Answer from the drawing. Dimensions are ordinates in mm from the lowest x, y and z of the part. Round coordinates to 2 decimals unless told otherwise and drop trailing zeros. Write each loop counter-clockwise with the first axis right and the second up, starting at its lowest first coordinate (ties: lowest second). Pieces come first, ordered by that corner, then holes. Notation, with made-up numbers: (69.25, -5.5) - (93.25, -5.5) arc R35 ccw to (93.25, 27.5) - close; hole circle Ø10 at (81, 62). An arc over 180 degrees is marked (long way). Answer as a JSON object with one key per item and string values.
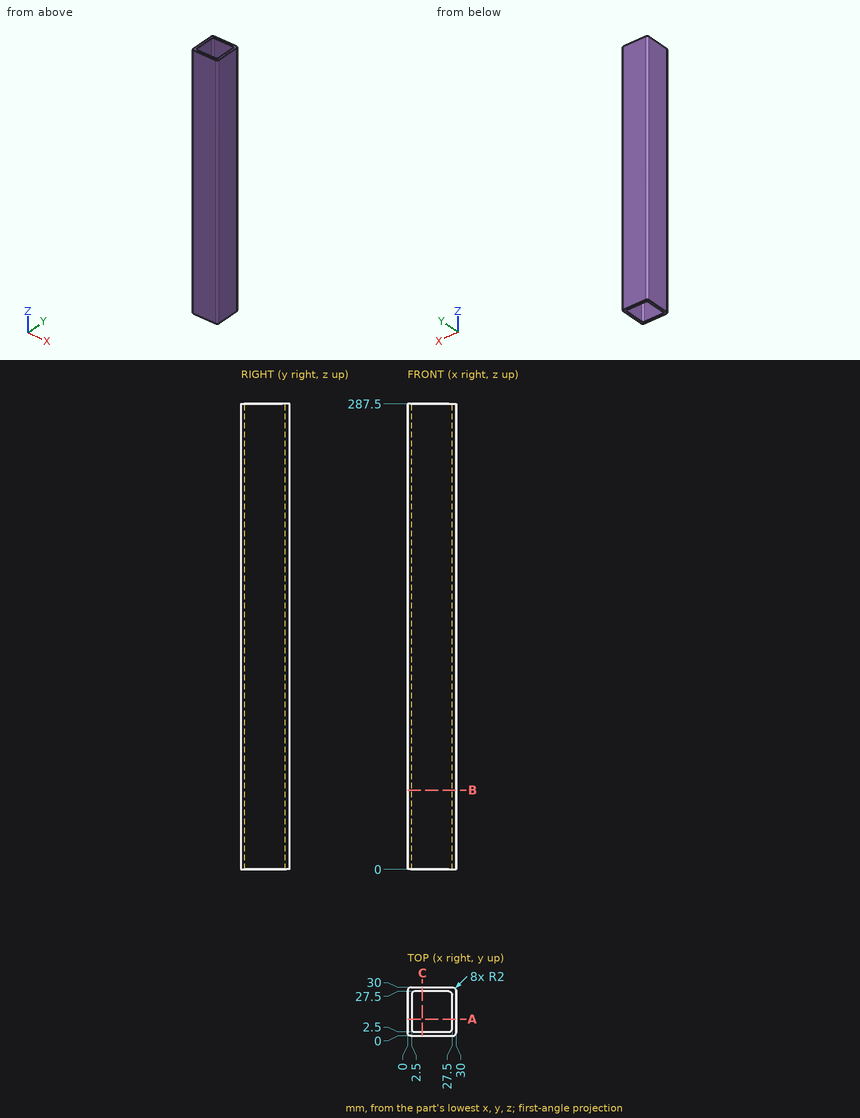
Item 1: A cutting plane is placed at A-A (y = 10.5). Write down the section's boundary in (x, z), and give its area (3 significant figures).
Results found:
{"outline": "(0, 0) - (2.5, 0) - (2.5, 287.5) - (0, 287.5) - close; (27.5, 0) - (30, 0) - (30, 287.5) - (27.5, 287.5) - close", "area": "1,440 mm²"}
Item 2: Each of these flat-tipped pins is pushed along its axis until it touches: P1, Ø1.5, axis at x = 4.5, y = 25.5, coming from the -Z side; P2, Ø4, axis at y = 19.5, z = 191.5, coming from the -X side. Where does it stop, or does it pass through?
Results found:
{"P1": "through", "P2": "x = 0"}
Item 3: A cutting plane is placed at B-B (z = 49). Write down the section's boundary in (x, y).
Results found:
{"outline": "(0, 2) arc R2 ccw to (2, 0) - (28, 0) arc R2 ccw to (30, 2) - (30, 28) arc R2 ccw to (28, 30) - (2, 30) arc R2 ccw to (0, 28) - close; hole (2.5, 4.5) arc R2 ccw to (4.5, 2.5) - (25.5, 2.5) arc R2 ccw to (27.5, 4.5) - (27.5, 25.5) arc R2 ccw to (25.5, 27.5) - (4.5, 27.5) arc R2 ccw to (2.5, 25.5) - close"}
Item 4: Consider line 1 along Y through (x, z) = (5, 60); line 2 along Y through (x, z) = (27.25, 140.5). Determine where each line is inside the solid, lowest interval first.
Results found:
{"line 1": "0 to 2.5, 27.5 to 30", "line 2": "0 to 3.53, 26.47 to 30"}
